from build123d import *

# Parameters (mm, degrees)
BOSS_EXTRUDE1_DEPTH               = 22
M12X1_25_TAPPED_HOLE1_D           = 10.8
M12X1_25_TAPPED_HOLE1_CSINK_D     = 12.05
M12X1_25_TAPPED_HOLE1_CSINK_ANGLE = 90


with BuildPart() as part:
    # Sketch1 → Boss-Extrude1 (new, symmetric)
    with BuildSketch(Plane.XY):
        Polygon((-38, 0), (-38, 10), (-27, 10), (-27, 6), (-25, 6), (-25, 15), (25, 15), (25, 6), (27, 6), (27, 10), (38, 10), (38, 0), align=None)
    extrude(amount=BOSS_EXTRUDE1_DEPTH, both=True)

    # M12x1.25 Tapped Hole1 (through all)
    with Locations(Plane(origin=(0, 15, 0), x_dir=(1, 0, 0), z_dir=(0, 1, 0))):
        with Locations((0, 0)):
            CounterSinkHole(M12X1_25_TAPPED_HOLE1_D / 2, M12X1_25_TAPPED_HOLE1_CSINK_D / 2, counter_sink_angle=M12X1_25_TAPPED_HOLE1_CSINK_ANGLE)


solid = part.part
Can you work these out from the model? Positions are in its coordinate system, mm. A direction names the side the tool comes from. Give positions to 0.01 mm unless a question says otherwise; leave off trailing zeros. Order: outer loops, then holes, each group sorted by start corner. A loop starts at its lowest first (then second) coordinate and runs counter-clockwise, first axis right, second up. Notation, with made-up numbers: M 78,70 L 99,70 A9 cw 99,77 Z; hole C 54.5,71.25 d6. An arc over 180 degrees is marked long. Use a Markdown table: item, result. Add a question column.
Item 1: Suppose I cut it at A-A (y = 7.25). List the corners of the cut face in (x, z) for me, then the cut area to 3 significant figures.
Item 2: If I drill on L1, parallel to Z at x = 0, y = 6; L2, parallel to X at y = 9, z = -6; L3, parallel to Y at x = -26.5, z = 12.5, over which ranges is the centre line in solid material (lowest first)? Write a range as [from, to].
Item 3: Suppose I cut it at D-D (y = 12.75). List the corners of the cut face in (x, z) for me.
Item 4: Suppose I cut it at C-C (z = 0). List the corners of the cut face in (x, y) for me (3 decimals).
Item 5: Suppose I cut it at B-B (x = 0). List the corners of the cut face in (y, z) for me (3 decimals).
Item 6: For faces 5 (the flat face through (32, 10, 0)), 6 (the flat face through (-25, 10, 0)), 7 (the flat face through (-33, 10, 0)), which set-ups out of +Z, -Z, +X, -X, +Y, -Y let a thin tool reach every point of the face, with its end or its side?
Item 7: We'd pull the mould along Z, two halves only. Please class faces 1 (the flat face through (-27, 8, 0)), 2 (the cylindrical face through (1.17, 7.09, 5.27)), 3 (the flat face through (1, 8, 22)), 4 (the flat face through (1, 8, -22)): +Z half, -Z half, draft (parallel to the pull), parting line (faces both ways), or undercut.
Item 8: Will these pins go through, and if not, where does the flat tip stop? pin 1 (0.6 mm diameter, centred on x = 26, z = 5.5, fed in from +Y); pin 2 (5.5 mm diameter, centred on x = 30, z = -8, fed in from +Y).
Answer sheet:
| question | item | result |
|---|---|---|
| 1 | outline | M -38,-22 L -27,-22 L -27,22 L -38,22 Z; M -25,-22 L 25,-22 L 25,22 L -25,22 Z; M 27,-22 L 38,-22 L 38,22 L 27,22 Z; hole C 0,0 d10.8 |
| 1 | area | 3,080 mm² |
| 2 | L1 | z = [-22, -5.4], [5.4, 22] |
| 2 | L2 | x = [-38, -27], [-25, 25], [27, 38] |
| 2 | L3 | y = [0, 6] |
| 3 | outline | M -25,-22 L 25,-22 L 25,22 L -25,22 Z; hole C 0,0 d10.8 |
| 4 | outline | M -38,0 L -5.4,0 L -5.4,14.375 L -6.025,15 L -25,15 L -25,6 L -27,6 L -27,10 L -38,10 Z; M 5.4,0 L 38,0 L 38,10 L 27,10 L 27,6 L 25,6 L 25,15 L 6.025,15 L 5.4,14.375 Z |
| 5 | outline | M 0,-22 L 15,-22 L 15,-6.025 L 14.375,-5.4 L 0,-5.4 Z; M 0,5.4 L 14.375,5.4 L 15,6.025 L 15,22 L 0,22 Z |
| 6 | face 5 | +Z, -Z, +X, +Y |
| 6 | face 6 | +Z, -Z, +Y |
| 6 | face 7 | +Z, -Z, -X, +Y |
| 7 | face 1 | draft |
| 7 | face 2 | undercut |
| 7 | face 3 | +Z half |
| 7 | face 4 | -Z half |
| 8 | pin 1 | stops at y = 6 |
| 8 | pin 2 | stops at y = 10 |
